Build history of the part. All positions in model axes, mm. A direction names the side the tool comes from. Round coordinates to 2 decimals unless told otherwise and drop trailing zeros. Order: outer loops, then holes, each group sorted by start corner. A loop starts at its lowest first (then second) coordinate and runs counter-clockwise, first axis right, second up. Notation, with made-up numbers: M -9.75,68 L 27.25,68 A15 cw 27.25,90 Z; hole C 84.25,8 d2. An arc over 180 degrees is marked long. Use CSV: the item, a comma, the result in double quotes.
from build123d import *

# Parameters (mm, degrees)
SKETCH1_R                  = 13
BOSS_EXTRUDE1_DEPTH        = 20
F_5_0MM_DOWEL_HOLE1_D      = 5
F_5_0MM_DOWEL_HOLE2_REACH  = 228.164
F_5_0MM_DOWEL_HOLE2_BORE_R = 2.5


with BuildPart() as part:
    # Sketch1 → Boss-Extrude1 (new body)
    with BuildSketch(Plane.XY):
        with BuildLine():
            Line((-57.251461988, 0), (52.748538012, 0))
            Line((52.748538012, 0), (52.748538012, 150))
            ThreePointArc((52.748538012, 150), (-2.251461988, 205), (-57.251461988, 150))
            Line((-57.251461988, 150), (-57.251461988, 0))
        make_face()
        with Locations((-2.251461988, 150)):
            Circle(SKETCH1_R, mode=Mode.SUBTRACT)
    extrude(amount=BOSS_EXTRUDE1_DEPTH)

    # Ø5.0mm Dowel Hole1 (through all)
    with Locations(Plane(origin=(-2.251461988, 190, 20), x_dir=(1, 0, 0), z_dir=(0, 0, 1))):
        with Locations((0, 0), (40, -40), (0, -80), (-40, -40)):
            Hole(F_5_0MM_DOWEL_HOLE1_D / 2)

    # Ø5.0mm Dowel Hole2 bore (on position points) → Ø5.0mm Dowel Hole2 (cut, up to next)
    with BuildSketch(Plane(origin=(-42.251461988, 0, 10), x_dir=(0, 0, -1), z_dir=(0, -1, 0)), mode=Mode.PRIVATE) as f_5_0mm_dowel_hole2_sk1:
        Circle(F_5_0MM_DOWEL_HOLE2_BORE_R)
    f_5_0mm_dowel_hole2_tool1 = extrude(f_5_0mm_dowel_hole2_sk1.sketch, amount=-F_5_0MM_DOWEL_HOLE2_REACH, mode=Mode.PRIVATE) & part.part
    # Ø5.0mm Dowel Hole2 bore (on position points) → Ø5.0mm Dowel Hole2 (cut, up to next)
    with BuildSketch(Plane(origin=(-42.251461988, 0, 10), x_dir=(0, 0, -1), z_dir=(0, -1, 0)), mode=Mode.PRIVATE) as f_5_0mm_dowel_hole2_sk2:
        with Locations((0, 80)):
            Circle(F_5_0MM_DOWEL_HOLE2_BORE_R)
    f_5_0mm_dowel_hole2_tool2 = extrude(f_5_0mm_dowel_hole2_sk2.sketch, amount=-F_5_0MM_DOWEL_HOLE2_REACH, mode=Mode.PRIVATE) & part.part
    add(f_5_0mm_dowel_hole2_tool1.solids().sort_by_distance((-42.251462, 0, 10))[0], mode=Mode.SUBTRACT)
    add(f_5_0mm_dowel_hole2_tool2.solids().sort_by_distance((37.748538, 0, 10))[0], mode=Mode.SUBTRACT)


solid = part.part
(1) Tool access for faces 5 (the face through (35.3, 74, 10.5)), 6 (the face through (-5.07, 137.31, 9.86)): list every direction of +Z, -Z, +X, -X, +Y, -Y with a clear straight run to the whole face (end or side of a thin tool).
Answer block:
face 5,"-Y"
face 6,"+Z, -Z"
(2) Cut at B-B, the plane z = 3.75. Give the cut face in (x, y), and give its area (3 significant figures).
Answer block:
outline,"M -57.25,0 L 52.75,0 L 52.75,150 A55 ccw -57.25,150 Z; hole C -42.25,150 d5; hole C -2.25,150 d26; hole C -2.25,110 d5; hole C -2.25,190 d5; hole C 37.75,150 d5"
area,"20,600 mm²"
(3) Cut at A-A, the plane x = -10.5. Give the cut face in (y, z), and give its area (3 significant figures).
Answer block:
outline,"M 0,0 L 139.95,0 L 139.95,20 L 0,20 Z; M 160.05,0 L 204.38,0 L 204.38,20 L 160.05,20 Z"
area,"3,690 mm²"
(4) Cut at C-C, the plane y = 110. Give the cut face in (x, z), and give its area (3 significant figures).
Answer block:
outline,"M -57.25,0 L -4.75,0 L -4.75,20 L -57.25,20 Z; M 0.25,0 L 52.75,0 L 52.75,20 L 0.25,20 Z; hole C -42.25,10 d5; hole C 37.75,10 d5"
area,"2,060 mm²"
(5) Two-plate mould, pull along X, no slides. Class faces 1 (the face through (-40.56, 73.95, 11.84)), 2 (the face through (-1.93, 192.48, 9.86)), 3 (the face through (52.749, 74, 10)), 4 (the face through (-3, 0, 10)): released by +X, released by -X, zero draft, split by the parting line, or undercut.
Answer block:
face 1,"undercut"
face 2,"undercut"
face 3,"released by +X"
face 4,"zero draft"
(6) Cut at D-D, the plane y = 190. Give the cut face in (x, z).
Answer block:
outline,"M -40,0 L -4.75,0 L -4.75,20 L -40,20 Z; M 0.25,0 L 35.5,0 L 35.5,20 L 0.25,20 Z"
(7) Wall check: line 1 (Y direction, x = -2.5, z = 13.25); line 2 (X direction, y = 43.5, z = 12); line 3 (Z direction, x = 38, y = 67). Give the ranges that are in metal, low to high. Write a range as from..to.
Answer block:
line 1,"y = 0..107.51, 112.49..137, 163..187.51, 192.49..205"
line 2,"x = -57.25..-43.75, -40.75..36.25, 39.25..52.75"
line 3,"z = 0..7.51, 12.49..20"
(8) Drop flat-ended pins along their axis: pin 1 (12 mm diameter, centred on x = 13.5, y = 61, fed in from -Z); pin 2 (3 mm diameter, centred on x = -2.25, y = 110, fed in from +Z); pin 3 (4.5 mm diameter, centred on x = -42.25, z = 10, fed in from -Y); pin 4 (4 mm diameter, centred on x = 37.75, z = 10, fed in from +Y). Give the stop position or say it passes through.
Answer block:
pin 1,"stops at z = 0"
pin 2,"passes through"
pin 3,"stops at y = 151.09"
pin 4,"stops at y = 189.76"
